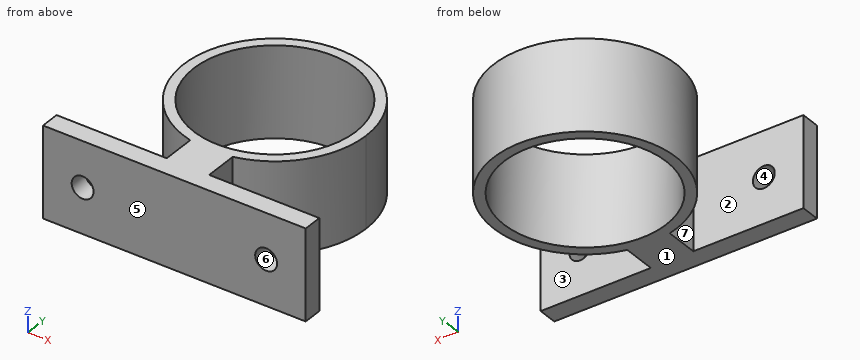
```python
from build123d import *

# Parameters (mm, degrees)
F0_R     = 14.097
F0_W     = 7.3929424398
F0_H     = 1.651
F1_DEPTH = 15.748
F2_R     = 1.905
F3_DEPTH = 9.4742


with BuildPart() as f1:
    # F0 (on Top) → F1 (new body)
    with BuildSketch(Plane.XY):
        with BuildLine():
            ThreePointArc((3.6964712199, -15.4386439016), (12.4638899549, -9.8319414254), (15.875, 0))
            ThreePointArc((15.875, 0), (-9.8319414254, 12.4638899549), (-3.6964712199, -15.4386439016))
            Line((-3.6964712199, -15.4386439016), (-3.6964712199, -15.1949884841))
            Line((-3.6964712199, -15.1949884841), (3.6964712199, -15.1949884841))
            Line((3.6964712199, -15.1949884841), (3.6964712199, -15.4386439016))
        make_face()
        Circle(F0_R, mode=Mode.SUBTRACT)
        with BuildLine():
            Line((-3.6964712199, -15.1949884841), (-3.6964712199, -15.4386439016))
            ThreePointArc((-3.6964712199, -15.4386439016), (0, -15.875), (3.6964712199, -15.4386439016))
            Line((3.6964712199, -15.4386439016), (3.6964712199, -15.1949884841))
            Line((3.6964712199, -15.1949884841), (-3.6964712199, -15.1949884841))
        make_face()
        with BuildLine():
            ThreePointArc((3.6964712199, -15.4386439016), (0, -15.875), (-3.6964712199, -15.4386439016))
            Line((-3.6964712199, -15.4386439016), (-3.6964712199, -21.1639884841))
            Line((-3.6964712199, -21.1639884841), (3.6964712199, -21.1639884841))
            Line((3.6964712199, -21.1639884841), (3.6964712199, -15.4386439016))
        make_face()
        with Locations((0, -21.9894884841)):
            Rectangle(F0_W, F0_H)
        Polygon((-3.6964712199, -22.8149884841), (-3.6964712199, -21.1639884841), (-22.86, -21.1639884841), (-22.86, -24.4659884841), (22.86, -24.4659884841), (22.86, -21.1639884841), (3.6964712199, -21.1639884841), (3.6964712199, -22.8149884841), align=None)
    extrude(amount=F1_DEPTH)

    # F2 (on face) → F3 (cut)
    with BuildSketch(Plane.XZ.offset(24.4659884841)):
        with Locations((-15.9683022648, 7.874)):
            Circle(F2_R)
        with Locations((15.9683022648, 7.874)):
            Circle(F2_R)
    extrude(amount=-F3_DEPTH, mode=Mode.SUBTRACT)


solid = f1.part
```
CAD build for the part. Positions are in the model's coordinates, mm. Face numbers are marked on the shaded views. A direction names the side the tool comes from. Coordinates: 2 decimals unless noted, no trailing zeros. Loops run counter-clockwise (first coordinate to the right, second up) from the corner with the lowest first, then second, coordinate; pieces in that order, holes last. Notation, with made-up numbers: (57.25, 76.5) - (89.25, 76.5) arc R27 cw to (89.25, 111.5) - close; hole circle Ø10 at (30, 55). An arc over 180 degrees is marked (long way). Use CSV: the item, a comma, the result in double quotes. Start each with the question number.
Q1. Drop flat-ended pins along their axis: P1, Ø6, axis at x = -7.5, y = -5.5, coming from the -Z side; P2, Ø1.7, axis at y = -19.5, z = 6, coming from the +X side; P3, Ø2, axis at x = 6.5, z = 8.5, coming from the +Y side; P4, Ø2, axis at y = -3.5, z = 10.5, coming from the +X side. Give the stop position or say it passes through.
Q2. 3-axis set-ups, long thin cutter, end or side, ignore diameter. For the marked faces 1, 2 and 3: which of +Z, -Z, +X, -X, +Y, -Y reach the whole face in a straight line?
Q3. Probe probe 1 along Y at (x, z) = (7, 14.75); probe 2 along Y at (x, z) = (6, 2.75); probe 3 along Y at (x, z) = (18.5, 13.5). List the from-to ranges inside material, lowest first. Write a range as from..to.
Q4. Two-plate mould, pull along X, no slides. Class the marked faces 4, 5, 6 and 7: +X half, -X half, draft (parallel to the pull), parting line (faces both ways), or undercut.
Q5. Cut at D-D, the plane y = 9. List the corners of the cut face in (x, z), then the cut area to 3 significant figures.
Q6. Cut at A-A, the plane z = 6.75. List the corners of the cut face in (x, y) (3 decimals).
Q7. Cut at C-C, the plane z = 1.5. List the corners of the cut face in (x, y) (3 decimals).
Q8. Cut at B-B, the plane x = -5. List the corners of the cut face in (y, z), then the cut area to 3 significant figures.
Here are the results:
1,P1,"through"
1,P2,"x = 3.7"
1,P3,"y = 14.89"
1,P4,"x = 15.68"
2,face 1,"-Z, +X, -X, +Y, -Y"
2,face 2,"+Z, -Z, -X"
2,face 3,"+Z, -Z, +X"
3,probe 1,"-24.47..-21.16, -14.25..-12.24, 12.24..14.25"
3,probe 2,"-24.47..-21.16, -14.7..-12.76, 12.76..14.7"
3,probe 3,"-24.47..-21.16"
4,face 4,"undercut"
4,face 5,"draft"
4,face 6,"undercut"
4,face 7,"-X half"
5,outline,"(-13.08, 0) - (-10.85, 0) - (-10.85, 15.75) - (-13.08, 15.75) - close; (10.85, 0) - (13.08, 0) - (13.08, 15.75) - (10.85, 15.75) - close"
5,area,"70.1 mm2"
6,outline,"(-22.86, -24.466) - (-17.506, -24.466) - (-17.506, -21.164) - (-22.86, -21.164) - close; (-14.43, -24.466) - (14.43, -24.466) - (14.43, -21.164) - (3.696, -21.164) - (3.696, -15.439) arc R15.875 ccw (long way) to (-3.696, -15.439) - (-3.696, -21.164) - (-14.43, -21.164) - close; (17.506, -24.466) - (22.86, -24.466) - (22.86, -21.164) - (17.506, -21.164) - close; hole circle Ø28.194 at (0, 0)"
7,outline,"(-22.86, -24.466) - (22.86, -24.466) - (22.86, -21.164) - (3.696, -21.164) - (3.696, -15.439) arc R15.875 ccw (long way) to (-3.696, -15.439) - (-3.696, -21.164) - (-22.86, -21.164) - close; hole circle Ø28.194 at (0, 0)"
8,outline,"(-24.47, 0) - (-21.16, 0) - (-21.16, 15.75) - (-24.47, 15.75) - close; (-15.07, 0) - (-13.18, 0) - (-13.18, 15.75) - (-15.07, 15.75) - close; (13.18, 0) - (15.07, 0) - (15.07, 15.75) - (13.18, 15.75) - close"
8,area,"111 mm2"
